```python
from build123d import *

# Parameters (mm, degrees)
SKETCH1_W           = 10
SKETCH1_H           = 10
BOSS_EXTRUDE1_DEPTH = 90
SKETCH2_W           = 8
SKETCH2_H           = 8
BOSS_EXTRUDE2_DEPTH = 80
SKETCH3_W           = 8
SKETCH3_H           = 8
BOSS_EXTRUDE3_DEPTH = 80
CUT_EXTRUDE1_DEPTH  = 0.6
CUT_EXTRUDE2_DEPTH  = 0.6
CUT_EXTRUDE3_DEPTH  = 0.6
CHAMFER1_SIZE       = 0.5


with BuildPart() as part:
    # Sketch1 → Boss-Extrude1 (new body)
    with BuildSketch(Plane.XY):
        with Locations((5, 5)):
            Rectangle(SKETCH1_W, SKETCH1_H)
    extrude(amount=BOSS_EXTRUDE1_DEPTH)

    # Sketch2 → Boss-Extrude2 (add)
    with BuildSketch(Plane(origin=(10, 0, 0), x_dir=(0, 0, -1), z_dir=(1, 0, 0))):
        with Locations((-4, 4)):
            Rectangle(SKETCH2_W, SKETCH2_H)
    extrude(amount=BOSS_EXTRUDE2_DEPTH)

    # Sketch3 → Boss-Extrude3 (add)
    with BuildSketch(Plane(origin=(0, 10, 0), x_dir=(1, 0, 0), z_dir=(0, 1, 0))):
        with Locations((4, -4)):
            Rectangle(SKETCH3_W, SKETCH3_H)
    extrude(amount=BOSS_EXTRUDE3_DEPTH)

    # Sketch6 → Cut-Extrude1 (cut)
    with BuildSketch(Plane(origin=(90, 0, 0), x_dir=(0, 0, -1), z_dir=(1, 0, 0))):
        Polygon((-5.923065511, 5.863746423), (-5.923065511, 5.39770075), (-4.082320318, 4.219515654), (-5.923065511, 3.041330558), (-5.923065511, 2.575284885), (-3.718137626, 3.986042096), (-1.423065511, 2.517592577), (-1.423065511, 2.98363825), (-3.353954934, 4.219515654), (-1.423065511, 5.455393058), (-1.423065511, 5.921438731), (-3.718137626, 4.452087769), align=None)
    extrude(amount=-CUT_EXTRUDE1_DEPTH, mode=Mode.SUBTRACT)

    # Sketch7 → Cut-Extrude2 (cut)
    with BuildSketch(Plane(origin=(0, 90, 0), x_dir=(0, 0, -1), z_dir=(0, 1, 0))):
        Polygon((-5.865477289, -5.670481901), (-5.865477289, -5.208041997), (-3.931883539, -4.025349689), (-5.865477289, -2.844460266), (-5.865477289, -2.382020363), (-3.504599885, -3.824328055), (-1.365477289, -3.824328055), (-1.365477289, -4.228174209), (-3.504599885, -4.228174209), align=None)
    extrude(amount=-CUT_EXTRUDE2_DEPTH, mode=Mode.SUBTRACT)

    # Sketch8 → Cut-Extrude3 (cut)
    with BuildSketch(Plane.XY.offset(90)):
        Polygon((3.422101108, 3.999142166), (2.960562647, 3.999142166), (2.960562647, 6.364526781), (6.999024185, 4.476906589), (6.999024185, 6.306834473), (7.460562647, 6.306834473), (7.460562647, 3.826065243), (3.422101108, 5.713685435), align=None)
    extrude(amount=-CUT_EXTRUDE3_DEPTH, mode=Mode.SUBTRACT)

    # Chamfer1
    chamfer1_edges = [part.edges().sort_by_distance(p)[0] for p in [
        (5.441331878, 4.769875339, 90),
        (7.460562647, 5.066449858, 90),
        (7.229793416, 6.306834473, 90),
        (6.999024185, 5.391870531, 90),
        (4.979793416, 5.420716685, 90),
        (2.960562647, 5.181834473, 90),
        (3.191331878, 3.999142166, 90),
        (3.422101108, 4.8564138, 90),
        (5, 10, 90),
        (10, 5, 90),
        (5, 0, 90),
        (0, 5, 90),
        (4.026251132, 90, 1.365477289),
        (3.824328055, 90, 2.435038587),
        (3.103174209, 90, 4.685038587),
        (2.613240314, 90, 5.865477289),
        (3.434904978, 90, 4.898680414),
        (4.616695843, 90, 4.898680414),
        (5.439261949, 90, 5.865477289),
        (4.949328055, 90, 4.685038587),
        (4.228174209, 90, 2.435038587),
        (90, 5.630723587, 5.923065511),
        (90, 4.808608202, 5.002692915),
        (90, 3.630423106, 5.002692915),
        (90, 2.808307721, 5.923065511),
        (90, 3.28066349, 4.820601568),
        (90, 3.251817337, 2.570601568),
        (90, 2.750615413, 1.423065511),
        (90, 3.601576952, 2.388510222),
        (90, 4.837454356, 2.388510222),
        (90, 5.688415894, 1.423065511),
        (90, 5.18676325, 2.570601568),
        (90, 5.157917096, 4.820601568),
        (8, 90, 4),
        (4, 90, 8),
        (0, 90, 4),
        (90, 4, 8),
        (90, 8, 4),
        (90, 0, 4),
        (45, 0, 0),
        (90, 4, 0),
        (50, 8, 0),
        (10, 9, 0),
        (9, 10, 0),
        (8, 50, 0),
        (4, 90, 0),
        (0, 45, 0),
    ]]
    chamfer(chamfer1_edges, length=CHAMFER1_SIZE)


solid = part.part
```
Verification items for the finished model (mm, model axes). A direction names the side the tool comes from. Give positions to 0.01 mm unless a question says otherwise; leave off trailing zeros. Loops run counter-clockwise (first coordinate to the right, second up) from the corner with the lowest first, then second, coordinate; pieces in that order, holes last. Notation, with made-up numbers: M 29,11.25 L 51,11.25 A25 ccw 51,44.25 Z; hole C 48,18.5 d7. An arc over 180 degrees is marked long. Return JSON: item names as keys, results as strings.
1) Mould release check, pull along Y, two halves, no side actions. Record for faces 1 (the flat face through (89.746, 5.654, 2.297)), 2 (the flat face through (90, 4, 6)), 3 (the flat face through (3.8, 89.4, 3.9)): released by +Y, released by -Y, zero draft, split by the parting line, or undercut.
Findings:
{"face 1": "undercut", "face 2": "zero draft", "face 3": "released by +Y"}
2) Material ranges on L1, parallel to Z at x = 43.5, y = 4; L2, parallel to Y at x = 4.5, z = 37, recorded low to high. Write a range as [from, to].
Findings:
{"L1": "z = [0, 8]", "L2": "y = [0, 10]"}
3) Gauge pin test, flat ends, axial feed: P1, Ø8, axis at x = 3, z = 56, coming from the +Y side; P2, Ø4, axis at x = 58.5, z = 5.5, coming from the +Y side; P3, Ø2.5, axis at x = 33, y = 2.5, coming from the +Z side. Record the tip position at first contact, or that the pin passes through.
Findings:
{"P1": "stops at y = 10", "P2": "stops at y = 8", "P3": "stops at z = 8"}
4) Tool access check on faces 4 (the flat face through (5.73, 4.36, 89.75)), 5 (the flat face through (49, 8, 4)), 6 (the flat face through (4, 49, 8)). Record the directions out of +Z, -Z, +X, -X, +Y, -Y that give a thin tool (end or side, any length) a straight path to the whole face; none if there is none.
Findings:
{"face 4": "+Z", "face 5": "+Z, -Z, +X, +Y", "face 6": "+Z, +X, -X, +Y"}
5) Section check C-C, the plane z = 33. Enter the section's corners in (x, y), and give its area (3 significant figures).
Findings:
{"outline": "M 0,0 L 10,0 L 10,10 L 0,10 Z", "area": "100 mm2"}
6) Section check A-A, the plane x = 27. Enter the section's corners in (y, z), and give its area (4 significant figures).
Findings:
{"outline": "M 0,0.5 L 0.5,0 L 7.5,0 L 8,0.5 L 8,8 L 0,8 Z", "area": "63.75 mm2"}
